from build123d import *

# Parameters (mm, degrees)
ESBO_O1_W                = 75
ESBO_O1_H                = 56
RESSALTO_EXTRUS_O1_DEPTH = 2
ESBO_O3_W                = 75
ESBO_O3_H                = 17
RESSALTO_EXTRUS_O3_DEPTH = 2
CORTE_EXTRUS_O1_REACH    = 4
ESBO_O4_R                = 2.5
CORTE_EXTRUS_O2_REACH    = 62
ESBO_O5_R                = 2.5
ESBO_O6_R                = 2.5
CORTE_EXTRUS_O3_DEPTH    = 2
CUT_EXTRUDE1_REACH       = 62
SKETCH1_R                = 2.5
CUT_EXTRUDE2_REACH       = 62
SKETCH2_R                = 2.5


with BuildPart() as part:
    # Esboço1 → Ressalto-extrusão1 (new body)
    with BuildSketch(Plane(origin=(0, 0, 0), x_dir=(1, 0, 0), z_dir=(0, 1, 0))):
        Rectangle(ESBO_O1_W, ESBO_O1_H)
    extrude(amount=RESSALTO_EXTRUS_O1_DEPTH)

    # Esboço3 → Ressalto-extrusão3 (add)
    with BuildSketch(Plane.XY.offset(28)):
        with Locations((0, 8.5)):
            Rectangle(ESBO_O3_W, ESBO_O3_H)
    ressalto_extrus_o3 = extrude(amount=RESSALTO_EXTRUS_O3_DEPTH)

    # Espelhar2: Ressalto-extrusão3 across plane
    add(ressalto_extrus_o3.mirror(Plane.XY))

    # Esboço4 → Corte-extrusão1 (cut, up to next)
    with BuildSketch(Plane(origin=(0, 0, 28), x_dir=(-1, 0, 0), z_dir=(0, 0, -1)), mode=Mode.PRIVATE) as corte_extrus_o1_sk1:
        with Locations((-7.575, 11.5)):
            Circle(ESBO_O4_R)
    corte_extrus_o1_tool1 = extrude(corte_extrus_o1_sk1.sketch, amount=-CORTE_EXTRUS_O1_REACH, mode=Mode.PRIVATE) & part.part
    add(corte_extrus_o1_tool1.solids().sort_by_distance((7.575, 11.5, 28))[0], mode=Mode.SUBTRACT)

    # Esboço5 → Corte-extrusão2 (cut, up to next)
    with BuildSketch(Plane.XY.offset(30), mode=Mode.PRIVATE) as corte_extrus_o2_sk1:
        with Locations((-27.5, 11.5)):
            Circle(ESBO_O5_R)
    corte_extrus_o2_tool1 = extrude(corte_extrus_o2_sk1.sketch, amount=-CORTE_EXTRUS_O2_REACH, mode=Mode.PRIVATE) & part.part
    add(corte_extrus_o2_tool1.solids().sort_by_distance((-27.5, 11.5, 30))[0], mode=Mode.SUBTRACT)

    # Esboço6 → Corte-extrusão3 (cut)
    with BuildSketch(Plane(origin=(0, 2, 0), x_dir=(1, 0, 0), z_dir=(0, 1, 0))):
        with Locations((-12.5, -14.5)):
            Circle(ESBO_O6_R)
        with Locations((27.5, -14.5)):
            Circle(ESBO_O6_R)
    extrude(amount=-CORTE_EXTRUS_O3_DEPTH, mode=Mode.SUBTRACT)

    # Sketch1 → Cut-Extrude1 (cut, up to next)
    with BuildSketch(Plane(origin=(0, 0, -30), x_dir=(-1, 0, 0), z_dir=(0, 0, -1)), mode=Mode.PRIVATE) as cut_extrude1_sk1:
        with Locations((-7.575, 9.5)):
            Circle(SKETCH1_R)
    cut_extrude1_tool1 = extrude(cut_extrude1_sk1.sketch, amount=-CUT_EXTRUDE1_REACH, mode=Mode.PRIVATE) & part.part
    add(cut_extrude1_tool1.solids().sort_by_distance((7.575, 9.5, -30))[0], mode=Mode.SUBTRACT)

    # Sketch2 → Cut-Extrude2 (cut, up to next)
    with BuildSketch(Plane(origin=(0, 0, -30), x_dir=(-1, 0, 0), z_dir=(0, 0, -1)), mode=Mode.PRIVATE) as cut_extrude2_sk1:
        with Locations((27.5, 9.5)):
            Circle(SKETCH2_R)
    cut_extrude2_tool1 = extrude(cut_extrude2_sk1.sketch, amount=-CUT_EXTRUDE2_REACH, mode=Mode.PRIVATE) & part.part
    add(cut_extrude2_tool1.solids().sort_by_distance((-27.5, 9.5, -30))[0], mode=Mode.SUBTRACT)


solid = part.part
Input: part model. Units: mm. Frame: model coordinates. A direction names the side the tool comes from. Coordinates: 2 decimals unless noted, no trailing zeros. Loops run counter-clockwise (first coordinate to the right, second up) from the corner with the lowest first, then second, coordinate; pieces in that order, holes last. Notation, with made-up numbers: (67, -10) -> (95, -10) arc R30 ccw to (95, 19) -> close; hole circle Ø10 at (81.25, 2). An arc over 180 degrees is marked (long way). Write item = value, one per line. Start each with the question number.
Item 1: Reachability of faces 5 (the face through (-28.04, 9.06, 29.01)), 6 (the face through (6.421, 7.282, -29.014)), 7 (the face through (-1, 10, 28)), 8 (the face through (-1, 9, 30)) from +Z, -Z, +X, -X, +Y, -Y: full face, straight path, thin tool, end or side. Return the list, or none.
Item 2: Cut plane D-D, the plane z = 25. Return loops of the section in (x, y).
Item 3: Material intervals for line 1 (X direction, y = 0.95, z = 14.5); line 2 (Z direction, x = 29.5, y = 7); line 3 (Z direction, x = 27.5, y = 0.5), sorted ascending.
Item 4: Cut plane C-C, the plane x = 19. Return loops of the section in (y, z), plus the area to 3 significant figures.
Item 5: Cut plane A-A, the plane z = 14.5. Return loops of the section in (x, y).
Item 6: Cut plane B-B, the plane x = -12.5. Return loops of the section in (y, z), plus the area to 3 significant figures.
Item 7: Mould query, pull axis X, two halves, no side actions, for faces 1 (the face through (-26.96, 7.06, -29.01)), 2 (the face through (37.5, 1.5, 0.1)), 3 (the face through (-1, 17, 29)), 4 (the face through (6.421, 9.282, 28.986)). Classes: pulls with the +X half, pulls with the -X half, needs draft (parallel to the pull), parting line crosses it, or undercut.
Item 8: First-contact query: P1, Ø3, axis at x = -12.5, z = 14.5, coming from the +Y side (3 decimals); P2, Ø6.5, axis at x = 27.5, z = 14.5, coming from the +Y side; P3, Ø4, axis at x = -27.5, y = 9.5, coming from the -Z side. Flat tips, straight axial feed; report the tip coordinate or a pass-through.
Ans:
q1.face_5 = +Z
q1.face_6 = -Z
q1.face_7 = +X, -X, +Y
q1.face_8 = +Z, +X, -X, +Y, -Y
q2.outline = (-37.5, 0) -> (37.5, 0) -> (37.5, 2) -> (-37.5, 2) -> close
q3.line_1 = -37.5 to -15, -10 to 25, 30 to 37.5
q3.line_2 = -30 to -28, 28 to 30
q3.line_3 = -30 to 12, 17 to 30
q4.outline = (0, -30) -> (17, -30) -> (17, -28) -> (2, -28) -> (2, 28) -> (17, 28) -> (17, 30) -> (0, 30) -> close
q4.area = 180 mm²
q5.outline = (-37.5, 0) -> (-15, 0) -> (-15, 2) -> (-37.5, 2) -> close; (-10, 0) -> (25, 0) -> (25, 2) -> (-10, 2) -> close; (30, 0) -> (37.5, 0) -> (37.5, 2) -> (30, 2) -> close
q6.outline = (0, -30) -> (17, -30) -> (17, -28) -> (2, -28) -> (2, 12) -> (0, 12) -> close; (0, 17) -> (2, 17) -> (2, 28) -> (17, 28) -> (17, 30) -> (0, 30) -> close
q6.area = 170 mm²
q7.face_1 = undercut
q7.face_2 = pulls with the +X half
q7.face_3 = needs draft
q7.face_4 = undercut
q8.P1 = through
q8.P2 = 2
q8.P3 = 28
